Source: three-view drawing plus pictorial views. Frame: mm from the lowest corner of the part. Coordinates: 2 decimals unless noted, no trailing zeros. Order: outer loops, then holes, each group sorted by start corner. A loop starts at its lowest first (then second) coordinate and runs counter-clockwise, first axis right, second up. Notation, with made-up numbers: (-5.5, 71) - (47.5, 71) arc R13 ccw to (47.5, 83) - close; hole circle Ø7 at (7, 37). An arc over 180 degrees is marked (long way). One line per question, with ' | ' between items.
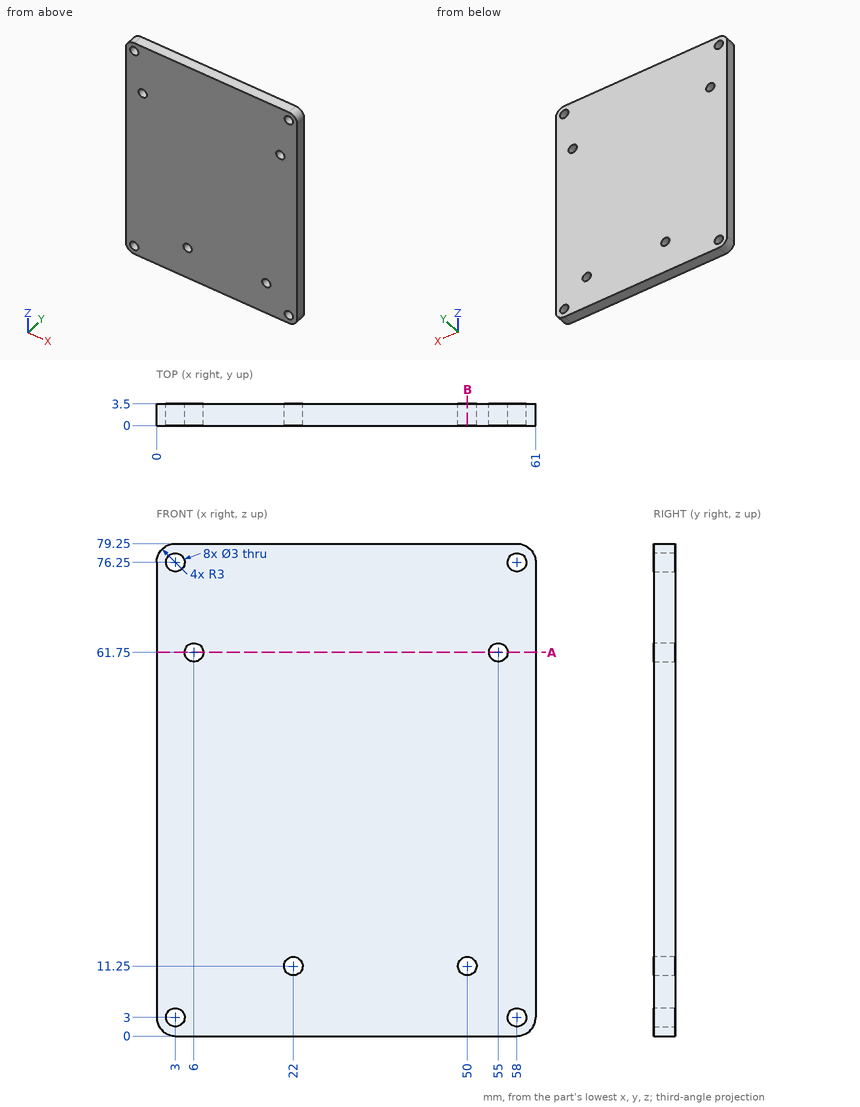
Item 1: Section A-A on z = 61.75. Return the cut outline in (x, y), and give its area (4 significant figures).
Data:
outline: (0, 0) - (4.5, 0) - (4.5, 3.5) - (0, 3.5) - close; (7.5, 0) - (53.5, 0) - (53.5, 3.5) - (7.5, 3.5) - close; (56.5, 0) - (61, 0) - (61, 3.5) - (56.5, 3.5) - close | area: 192.5 mm^2
Item 2: Section B-B on x = 50. Return the cut outline in (y, z).
Data:
outline: (0, 0) - (3.5, 0) - (3.5, 9.75) - (0, 9.75) - close; (0, 12.75) - (3.5, 12.75) - (3.5, 79.25) - (0, 79.25) - close
Item 3: Ray query, line 1 (X direction, y = 0.7, z = 61.75); line 2 (X direction, y = 1, z = 76.25); line 3 (Z direction, x = 56, y = 0.7). Return the intervals inside material, ascending.
Data:
line 1: 0 to 4.5, 7.5 to 53.5, 56.5 to 61 | line 2: 0 to 1.5, 4.5 to 56.5, 59.5 to 61 | line 3: 0 to 60.63, 62.87 to 79.25
